Geometry: see drawing. Coordinates: mm, zero at the bounding-box minimum. A direction names the side the tool comes from. Give positions to 0.01 mm unless a question says otherwise; leave off trailing zeros. Write each loop counter-clockwise with the first axis right and the second up, starting at its lowest first coordinate (ties: lowest second). Pieces come first, ordered by that corner, then holes. Notation, with made-up numbers: (-36, -8.5) -> (-10, -8.5) arc R32 ccw to (-10, 24.5) -> close; hole circle Ø10 at (-23, 48). An arc over 180 degrees is marked (long way). Write item = value, one per line.
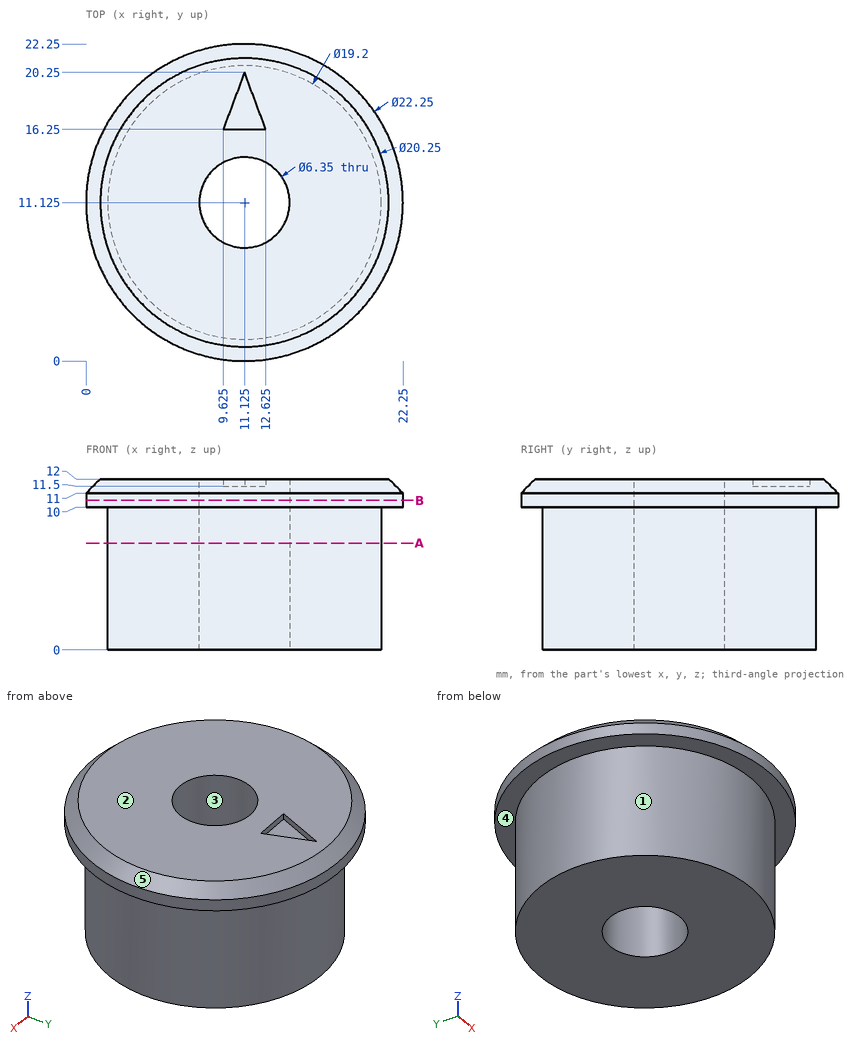
(1) First-contact query: pin 1 (0.6 mm diameter, centred on x = 11.5, z = 12, fed in from +Y); pin 2 (3.5 mm diameter, centred on x = 11, y = 18, fed in from +Z); pin 3 (3 mm diameter, centred on x = 7.5, z = 10.5, fed in from -Y); pin 4 (1 mm diameter, centred on y = 4, z = 2.5, fed in from +X). Flat tips, straight axial feed; report the tip coordinate or a pass-through.
Values follow:
pin_1 = 21.54
pin_2 = 12
pin_3 = 0.2
pin_4 = 18.07
(2) Access query for the marked faces 1 and 2. Directions: +Z, -Z, +X, -X, +Y, -Y. A direction counts if a zero-diameter tool reaches every point of the face in a straight line with its end or side. Return the directions, or none.
Values follow:
face_1 = -Z
face_2 = +Z, +X, -X, +Y, -Y
(3) Material intervals for line 1 (X direction, y = 12.75, z = 10.5); line 2 (X direction, y = 13, z = 3.75); line 3 (Y direction, x = 13.5, z = 6.5), sorted ascending.
Values follow:
line_1 = 0.12 to 8.4, 13.85 to 22.13
line_2 = 1.71 to 8.56, 13.69 to 20.54
line_3 = 1.82 to 9.02, 13.23 to 20.43
(4) Section query B-B (z = 10.5). Return loops of the section in (x, y) (3 decimals).
Values follow:
outline = circle Ø22.25 at (11.125, 11.125); hole circle Ø6.35 at (11.125, 11.125)
(5) Pull-direction query (Y, two-part tool) for the marked faces 3, 4 and 5; classes: pulls with the +Y half, pulls with the -Y half, needs draft (parallel to the pull), parting line crosses it, or undercut.
Values follow:
face_3 = undercut
face_4 = needs draft
face_5 = parting line crosses it
(6) Section query A-A (z = 7.5). Return loops of the section in (x, y) (3 decimals), plus the area to 3 significant figures.
Values follow:
outline = circle Ø19.2 at (11.125, 11.125); hole circle Ø6.35 at (11.125, 11.125)
area = 258 mm2
